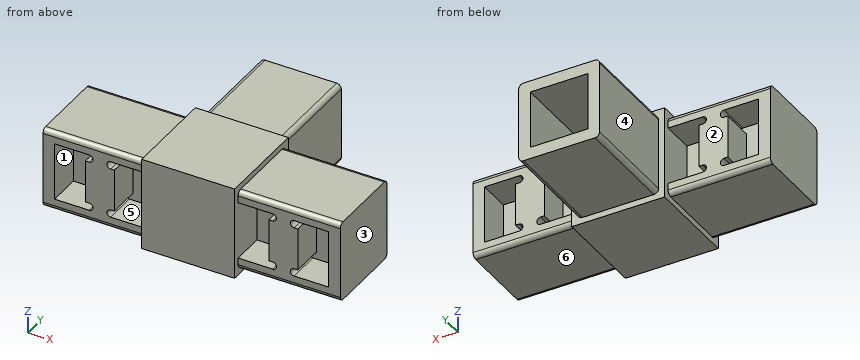
```python
from build123d import *

# Parameters (mm, degrees)
CUT_EXTRUDE1_START       = -25.4
CUT_EXTRUDE1_OUTLINE_W   = 81.28
CUT_EXTRUDE1_OUTLINE_H   = 22.098
CUT_EXTRUDE1_DEPTH       = 23.749
CUT_EXTRUDE1_START_2     = -1.651
CUT_EXTRUDE1_2_OUTLINE_W = 53.34
CUT_EXTRUDE1_2_OUTLINE_H = 22.098
CUT_EXTRUDE1_2_DEPTH     = 1.651
SKETCH2_W                = 27.94
SKETCH2_H                = 22.098
CUT_EXTRUDE2_DEPTH       = 1.651
SKETCH3_W                = 27.94
SKETCH3_H                = 22.098
CUT_EXTRUDE3_DEPTH       = 1.651
SKETCH4_W                = 27.94
SKETCH4_H                = 22.098
CUT_EXTRUDE4_DEPTH       = 1.651
SKETCH5_W                = 25.4
SKETCH5_H                = 25.4
BOSS_EXTRUDE1_DEPTH      = 1.651
SKETCH6_W                = 25.4
SKETCH6_H                = 25.4
BOSS_EXTRUDE2_DEPTH      = 1.651
CUT_EXTRUDE5_DEPTH       = 8.89
CUT_EXTRUDE6_DEPTH       = 8.89
CUT_EXTRUDE7_START       = -8.89
CUT_EXTRUDE7_DEPTH       = 8.89
CUT_EXTRUDE8_START       = -8.89
CUT_EXTRUDE8_DEPTH       = 8.89
CUT_EXTRUDE9_DEPTH       = 8.89
CUT_EXTRUDE10_START      = -8.89
CUT_EXTRUDE10_DEPTH      = 8.89
CUT_EXTRUDE11_DEPTH      = 8.89
CUT_EXTRUDE12_START      = -8.89
CUT_EXTRUDE12_DEPTH      = 8.89
SKETCH15_W               = 22.098
SKETCH15_H               = 22.098
BOSS_EXTRUDE3_DEPTH      = 27.94
SKETCH16_W               = 15.748
SKETCH16_H               = 15.748
CUT_EXTRUDE13_DEPTH      = 27.94
FILLET1_R                = 1.27


with BuildPart() as part:
    # Cut-Extrude1: read off the stored shape, not the designer's step
    # Cut-Extrude1 outline → Cut-Extrude1 (new body)
    with BuildSketch(Plane.XY.offset(12.7).offset(CUT_EXTRUDE1_START)):
        Rectangle(CUT_EXTRUDE1_OUTLINE_W, CUT_EXTRUDE1_OUTLINE_H)
    extrude(amount=CUT_EXTRUDE1_DEPTH)

    # Cut-Extrude1 2 outline → Cut-Extrude1 2 (add)
    with BuildSketch(Plane.XY.offset(12.7).offset(CUT_EXTRUDE1_START_2)):
        with Locations((13.97, 0)):
            Rectangle(CUT_EXTRUDE1_2_OUTLINE_W, CUT_EXTRUDE1_2_OUTLINE_H)
    extrude(amount=CUT_EXTRUDE1_2_DEPTH)

    # Sketch2 → Cut-Extrude2 (cut)
    with BuildSketch(Plane(origin=(0, 0, -12.7), x_dir=(-1, 0, 0), z_dir=(0, 0, -1))):
        with Locations((26.67, 0)):
            Rectangle(SKETCH2_W, SKETCH2_H)
    extrude(amount=-CUT_EXTRUDE2_DEPTH, mode=Mode.SUBTRACT)

    # Sketch3 → Cut-Extrude3 (cut)
    with BuildSketch(Plane(origin=(0, 0, -12.7), x_dir=(-1, 0, 0), z_dir=(0, 0, -1))):
        with Locations((-26.67, 0)):
            Rectangle(SKETCH3_W, SKETCH3_H)
    extrude(amount=-CUT_EXTRUDE3_DEPTH, mode=Mode.SUBTRACT)

    # Sketch4 → Cut-Extrude4 (cut)
    with BuildSketch(Plane.XY.offset(12.7)):
        with Locations((26.67, 0)):
            Rectangle(SKETCH4_W, SKETCH4_H)
    extrude(amount=-CUT_EXTRUDE4_DEPTH, mode=Mode.SUBTRACT)

    # Sketch5 → Boss-Extrude1 (add)
    with BuildSketch(Plane(origin=(0, 11.049, 0), x_dir=(-1, 0, 0), z_dir=(0, 1, 0))):
        Rectangle(SKETCH5_W, SKETCH5_H)
    extrude(amount=BOSS_EXTRUDE1_DEPTH)

    # Sketch6 → Boss-Extrude2 (add)
    with BuildSketch(Plane.XZ.offset(11.049)):
        Rectangle(SKETCH6_W, SKETCH6_H)
    extrude(amount=BOSS_EXTRUDE2_DEPTH)

    # Sketch7 → Cut-Extrude5 (cut)
    with BuildSketch(Plane(origin=(0, 11.049, 0), x_dir=(-1, 0, 0), z_dir=(0, 1, 0))):
        with BuildLine():
            Line((-12.7, -7.874), (-12.7, 7.874))
            Line((-12.7, 7.874), (-22.1615, 7.874))
            ThreePointArc((-22.1615, 7.874), (-23.1775, 6.858), (-22.1615, 5.842))
            Line((-22.1615, 5.842), (-21.1455, 5.842))
            Line((-21.1455, 5.842), (-21.1455, -5.842))
            Line((-21.1455, -5.842), (-22.1615, -5.842))
            ThreePointArc((-22.1615, -5.842), (-23.1775, -6.858), (-22.1615, -7.874))
            Line((-22.1615, -7.874), (-12.7, -7.874))
        make_face()
    extrude(amount=-CUT_EXTRUDE5_DEPTH, mode=Mode.SUBTRACT)

    # Sketch8 → Cut-Extrude6 (cut)
    with BuildSketch(Plane.XZ.offset(11.049)):
        with BuildLine():
            Line((-22.1615, 5.842), (-21.1455, 5.842))
            Line((-21.1455, 5.842), (-21.1455, -5.842))
            Line((-21.1455, -5.842), (-22.1615, -5.842))
            ThreePointArc((-22.1615, -5.842), (-23.1775, -6.858), (-22.1615, -7.874))
            Line((-22.1615, -7.874), (-12.7, -7.874))
            Line((-12.7, -7.874), (-12.7, 7.874))
            Line((-12.7, 7.874), (-22.1615, 7.874))
            ThreePointArc((-22.1615, 7.874), (-23.1775, 6.858), (-22.1615, 5.842))
        make_face()
    extrude(amount=-CUT_EXTRUDE6_DEPTH, mode=Mode.SUBTRACT)

    # Sketch9 → Cut-Extrude7 (cut)
    with BuildSketch(Plane.XZ.offset(11.049).offset(CUT_EXTRUDE7_START)):
        with BuildLine():
            Line((12.7, 7.874), (12.7, -7.874))
            Line((12.7, -7.874), (22.1615, -7.874))
            ThreePointArc((22.1615, -7.874), (23.1775, -6.858), (22.1615, -5.842))
            Line((22.1615, -5.842), (21.1455, -5.842))
            Line((21.1455, -5.842), (21.1455, 5.842))
            Line((21.1455, 5.842), (22.1615, 5.842))
            ThreePointArc((22.1615, 5.842), (23.1775, 6.858), (22.1615, 7.874))
            Line((22.1615, 7.874), (12.7, 7.874))
        make_face()
    extrude(amount=CUT_EXTRUDE7_DEPTH, mode=Mode.SUBTRACT)

    # Sketch10 → Cut-Extrude8 (cut)
    with BuildSketch(Plane(origin=(0, 11.049, 0), x_dir=(-1, 0, 0), z_dir=(0, 1, 0)).offset(CUT_EXTRUDE8_START)):
        with BuildLine():
            Line((21.1455, 5.842), (22.1615, 5.842))
            ThreePointArc((22.1615, 5.842), (23.1775, 6.858), (22.1615, 7.874))
            Line((22.1615, 7.874), (12.7, 7.874))
            Line((12.7, 7.874), (12.7, -7.874))
            Line((12.7, -7.874), (22.1615, -7.874))
            ThreePointArc((22.1615, -7.874), (23.1775, -6.858), (22.1615, -5.842))
            Line((22.1615, -5.842), (21.1455, -5.842))
            Line((21.1455, -5.842), (21.1455, 5.842))
        make_face()
    extrude(amount=CUT_EXTRUDE8_DEPTH, mode=Mode.SUBTRACT)

    # Sketch11 → Cut-Extrude9 (cut)
    with BuildSketch(Plane.XZ.offset(11.049)):
        with BuildLine():
            Line((28.0035, 5.842), (29.0195, 5.842))
            Line((29.0195, 5.842), (29.0195, -5.842))
            Line((29.0195, -5.842), (28.0035, -5.842))
            ThreePointArc((28.0035, -5.842), (26.9875, -6.858), (28.0035, -7.874))
            Line((28.0035, -7.874), (37.465, -7.874))
            Line((37.465, -7.874), (37.465, 7.874))
            Line((37.465, 7.874), (28.0035, 7.874))
            ThreePointArc((28.0035, 7.874), (26.9875, 6.858), (28.0035, 5.842))
        make_face()
    extrude(amount=-CUT_EXTRUDE9_DEPTH, mode=Mode.SUBTRACT)

    # Sketch12 → Cut-Extrude10 (cut)
    with BuildSketch(Plane(origin=(0, 11.049, 0), x_dir=(-1, 0, 0), z_dir=(0, 1, 0)).offset(CUT_EXTRUDE10_START)):
        with BuildLine():
            Line((-29.0195, -5.842), (-29.0195, 5.842))
            Line((-29.0195, 5.842), (-28.0035, 5.842))
            ThreePointArc((-28.0035, 5.842), (-26.9875, 6.858), (-28.0035, 7.874))
            Line((-28.0035, 7.874), (-37.465, 7.874))
            Line((-37.465, 7.874), (-37.465, -7.874))
            Line((-37.465, -7.874), (-28.0035, -7.874))
            ThreePointArc((-28.0035, -7.874), (-26.9875, -6.858), (-28.0035, -5.842))
            Line((-28.0035, -5.842), (-29.0195, -5.842))
        make_face()
    extrude(amount=CUT_EXTRUDE10_DEPTH, mode=Mode.SUBTRACT)

    # Sketch13 → Cut-Extrude11 (cut)
    with BuildSketch(Plane(origin=(0, 11.049, 0), x_dir=(-1, 0, 0), z_dir=(0, 1, 0))):
        with BuildLine():
            Line((28.0035, -7.874), (37.465, -7.874))
            Line((37.465, -7.874), (37.465, 7.874))
            Line((37.465, 7.874), (28.0035, 7.874))
            ThreePointArc((28.0035, 7.874), (26.9875, 6.858), (28.0035, 5.842))
            Line((28.0035, 5.842), (29.0195, 5.842))
            Line((29.0195, 5.842), (29.0195, -5.842))
            Line((29.0195, -5.842), (28.0035, -5.842))
            ThreePointArc((28.0035, -5.842), (26.9875, -6.858), (28.0035, -7.874))
        make_face()
    extrude(amount=-CUT_EXTRUDE11_DEPTH, mode=Mode.SUBTRACT)

    # Sketch14 → Cut-Extrude12 (cut)
    with BuildSketch(Plane.XZ.offset(11.049).offset(CUT_EXTRUDE12_START)):
        with BuildLine():
            Line((-37.465, 7.874), (-37.465, -7.874))
            Line((-37.465, -7.874), (-28.0035, -7.874))
            ThreePointArc((-28.0035, -7.874), (-26.9875, -6.858), (-28.0035, -5.842))
            Line((-28.0035, -5.842), (-29.0195, -5.842))
            Line((-29.0195, -5.842), (-29.0195, 5.842))
            Line((-29.0195, 5.842), (-28.0035, 5.842))
            ThreePointArc((-28.0035, 5.842), (-26.9875, 6.858), (-28.0035, 7.874))
            Line((-28.0035, 7.874), (-37.465, 7.874))
        make_face()
    extrude(amount=CUT_EXTRUDE12_DEPTH, mode=Mode.SUBTRACT)

    # Sketch15 → Boss-Extrude3 (add)
    with BuildSketch(Plane(origin=(0, 12.7, 0), x_dir=(-1, 0, 0), z_dir=(0, 1, 0))):
        Rectangle(SKETCH15_W, SKETCH15_H)
    extrude(amount=BOSS_EXTRUDE3_DEPTH)

    # Sketch16 → Cut-Extrude13 (cut)
    with BuildSketch(Plane(origin=(0, 40.64, 0), x_dir=(-1, 0, 0), z_dir=(0, 1, 0))):
        Rectangle(SKETCH16_W, SKETCH16_H)
    extrude(amount=-CUT_EXTRUDE13_DEPTH, mode=Mode.SUBTRACT)

    # Fillet1
    fillet1_edges = [part.edges().sort_by_distance(p)[0] for p in [
        (11.049, 26.67, 11.049),
        (-26.67, 11.049, 11.049),
        (-26.67, -11.049, -11.049),
        (26.67, 11.049, 11.049),
        (11.049, 26.67, -11.049),
        (26.67, 11.049, -11.049),
        (-26.67, -11.049, 11.049),
        (26.67, -11.049, 11.049),
        (-26.67, 11.049, -11.049),
        (-11.049, 26.67, 11.049),
        (26.67, -11.049, -11.049),
        (-11.049, 26.67, -11.049),
    ]]
    fillet(fillet1_edges, radius=FILLET1_R)


solid = part.part
```
Can you work these out from the model? Positions are in its coordinate system, mm. Face numbers are marked on the shaded views. A direction names the side the tool comes from. Coordinates: 2 decimals unless noted, no trailing zeros. Loops run counter-clockwise (first coordinate to the right, second up) from the corner with the lowest first, then second, coordinate; pieces in that order, holes last.
1) Which directions (+Z, -Z, +X, -X, +Y, -Y) give clear straight access to the entire face, cutting with the end or side of a thin tool? Please do the marked faces 4, 5 and 6.
2) Thinking about a two-plate mould opening in X: for the marked faces 1, 2 and 3, which applies, pulls with the +X half, pulls with the -X half, needs draft (parallel to the pull), parting line crosses it, or undercut?
3) I need wall thicknesses on probe 1 along X at (y, z) = (-7.5, 3.5) (1 decimal); probe 2 along X at (y, z) = (23, -7.75); probe 3 along Z at (x, y) = (-10, 17.5). Which ranges of each line are inside material? Lowest first, please.
4) Imagine slicing it at C-C on y = -1. List the corners of the cut face in (x, z) for me.
5) Imagine slicing it at B-B on x = -4.5. List the corners of the cut face in (y, z) for me, plus the area to 3 significant figures.
6) Imagine slicing it at A-A on y = 26.5. List the corners of the cut face in (x, z) for me, plus the area to 3 significant figures.
7) For pin 1 (5 mm diameter, centred on x = 20, z = 3.5, fed in from +Y); pin 2 (10 mm diameter, centred on x = -15.5, y = 5, fed in from +Z); pin 3 (5 mm diameter, centred on x = 24.5, z = 2.5, fed in from -Y); pin 4 (8 mm diameter, centred on y = 28, z = -2.5, fed in from -X), each with a flat end and sliding along its axis, tell me the tip position at first contact or that it passes through.
8) Imagine slicing it at D-D on x = 19. List the corners of the cut face in (y, z) for me.
Completed:
1. face 4: +Z, -Z, -X, +Y
1. face 5: -Y
1. face 6: -Z, +X, +Y, -Y
2. face 1: undercut
2. face 2: needs draft
2. face 3: pulls with the +X half
3. probe 1: x = -40.6 to -37.5, -29 to -21.1, -12.7 to 12.7, 21.1 to 29, 37.5 to 40.6
3. probe 2: x = -11.05 to -7.87, 7.87 to 11.05
3. probe 3: z = -11.03 to 11.03
4. outline: (-40.64, -11.05) - (-12.7, -11.05) - (-12.7, -12.7) - (12.7, -12.7) - (12.7, -11.05) - (40.64, -11.05) - (40.64, 11.05) - (12.7, 11.05) - (12.7, 12.7) - (-12.7, 12.7) - (-12.7, 11.05) - (-40.64, 11.05) - close
5. outline: (-12.7, -12.7) - (12.7, -12.7) - (12.7, -11.05) - (40.64, -11.05) - (40.64, -7.87) - (12.7, -7.87) - (12.7, 7.87) - (40.64, 7.87) - (40.64, 11.05) - (12.7, 11.05) - (12.7, 12.7) - (-12.7, 12.7) - close
5. area: 823 mm2
6. outline: (-11.05, -9.78) arc R1.27 ccw to (-9.78, -11.05) - (9.78, -11.05) arc R1.27 ccw to (11.05, -9.78) - (11.05, 9.78) arc R1.27 ccw to (9.78, 11.05) - (-9.78, 11.05) arc R1.27 ccw to (-11.05, 9.78) - close; hole (-7.87, -7.87) - (7.87, -7.87) - (7.87, 7.87) - (-7.87, 7.87) - close
6. area: 239 mm2
7. pin 1: stops at y = 11.05
7. pin 2: stops at z = 12.7
7. pin 3: stops at y = -11.05
7. pin 4: stops at x = -11.05
8. outline: (-11.05, -9.78) arc R1.27 ccw to (-9.78, -11.05) - (9.78, -11.05) arc R1.27 ccw to (11.05, -9.78) - (11.05, -7.87) - (2.16, -7.87) - (2.16, 7.87) - (11.05, 7.87) - (11.05, 9.78) arc R1.27 ccw to (9.78, 11.05) - (-9.78, 11.05) arc R1.27 ccw to (-11.05, 9.78) - (-11.05, 7.87) - (-2.16, 7.87) - (-2.16, -7.87) - (-11.05, -7.87) - close
